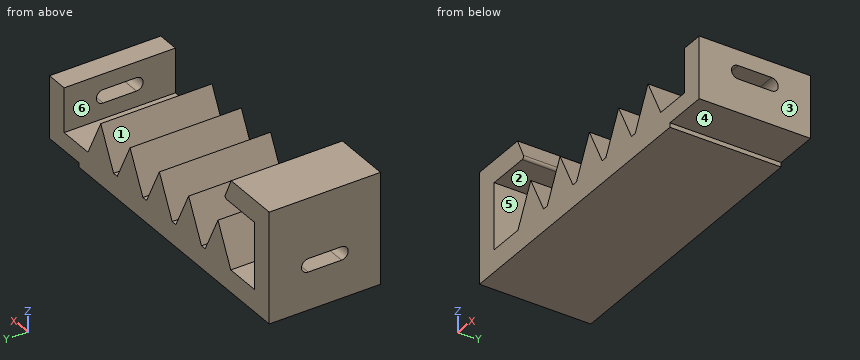
```python
from build123d import *

# Parameters (mm, degrees)
PAD028_DEPTH    = 2.5
POCKET033_DEPTH = 2


with BuildPart() as part:
    # Sketch063 → Pad028 (new body, symmetric)
    with BuildSketch(Plane.XZ):
        with BuildLine():
            Line((-7.5, 0), (-7.5, 5))
            Line((-7.5, 5), (-4.89997, 5))
            Line((-4.89997, 5), (-4.5, 4.142262))
            ThreePointArc((-4.590631, 4), (-4.506292, 4.04627), (-4.5, 4.142262))
            Line((-4.590631, 4), (-6.5, 4))
            Line((-6.5, 4), (-6.5, 1))
            Line((-6.5, 1), (-5, 1))
            Line((-4.875, 1), (-5, 1))
            Line((-4.875, 1), (-4, 2.75))
            Line((-4, 2.75), (-3.125, 1))
            Line((-3.125, 1), (-2.875, 1))
            Line((-2.875, 1), (-2, 2.75))
            Line((-2, 2.75), (-1.125, 1))
            Line((-1.125, 1), (-0.875, 1))
            Line((-0.875, 1), (0, 2.75))
            Line((0, 2.75), (0.875, 1))
            Line((0.875, 1), (1.125, 1))
            Line((1.125, 1), (2, 2.75))
            Line((2, 2.75), (2.875, 1))
            Line((2.875, 1), (3.125, 1))
            Line((3.125, 1), (4, 2.75))
            Line((4, 2.75), (4.875, 1))
            Line((4.875, 1), (5, 1))
            Line((5, 1), (6.5, 1))
            Line((6.5, 1), (6.5, 3))
            Line((6.5, 3), (7.5, 3))
            Line((7.5, 3), (7.5, 0.2))
            Line((5.5, 0.2), (7.5, 0.2))
            Line((5.5, 0), (5.5, 0.2))
            Line((5.5, 0), (-7.5, 0))
        make_face()
    extrude(amount=PAD028_DEPTH, both=True)

    # Sketch062 (on Face28 of Pad028) → Pocket033 (cut)
    with BuildSketch(Plane(origin=(7.5, 0, 0), x_dir=(0, 0, 1), z_dir=(1, 0, 0))):
        with BuildLine():
            ThreePointArc((2.3, 0.75), (2, 1.05), (1.7, 0.75))
            Line((1.7, 0.75), (1.7, -0.75))
            ThreePointArc((1.7, -0.75), (2, -1.05), (2.3, -0.75))
            Line((2.3, 0.75), (2.3, -0.75))
        make_face()
    pocket033 = extrude(amount=-POCKET033_DEPTH, mode=Mode.SUBTRACT)

    # Mirrored003: Pocket033 across YZ
    add(pocket033.mirror(Plane.YZ), mode=Mode.SUBTRACT)


solid = part.part
```
Can you work these out from the model? Positions are in its coordinate system, mm. Face numbers are marked on the shaded views. A direction names the side the tool comes from. Give positions to 0.01 mm unless a question says otherwise; leave off trailing zeros. Loops run counter-clockwise (first coordinate to the right, second up) from the corner with the lowest first, then second, coordinate; pieces in that order, holes last. Notation, with made-up numbers: M -34.75,-35 L 22.25,-35 A24 ccw 22.25,-14 Z; hole C 2,65.5 d4. An arc over 180 degrees is marked long. One line per question, with ' | ' between items. Start each with the question number.
Q1. If we section it at B-B (z = 1.4): Please give me the cut outline in (x, y) (3 decimals), plus the area to 4 significant figures.
Q2. If I drill on line 1 (Z direction, x = -5, y = 1.3); line 2 (Z direction, x = 6.75, y = 0.05); line 3 (X direction, y = 0.8, z = 3.7), over which ranges is the centre line in solid material (lowest first)? Write a range as from..to.
Q3. If we section it at A-A (x = -6.25): Please give me the cut outline in (y, z), plus the area to 3 significant figures.
Q4. For the marked faces 4, 5 and 6, which set-ups out of +Z, -Z, +X, -X, +Y, -Y let a thin tool reach every point of the face, with its end or its side?
Q5. For pin 1 Ø1.5 at (y, z) = (-0.5, 2) entering from +X; pin 2 Ø1.1 at (x, y) = (7, 0) entering from -Z, each with a flat end and sliding along its axis, tell me the tip position at first contact or that it passes through.
Q6. If we section it at C-C (y = 0.3): State how many separate pieces and enclosed holes the cut face has, plus the area to 3 significant figures.
Q7. If we mould it in two halves opening along X, with no side actions, what happens to the marked faces 1, 2 and 3? For each: +X half, -X half, draft (parallel to the pull), parting line (faces both ways), or undercut.
Computed:
1) outline: M -7.5,-2.5 L -6.5,-2.5 L -6.5,2.5 L -7.5,2.5 Z; M -4.675,-2.5 L -3.325,-2.5 L -3.325,2.5 L -4.675,2.5 Z; M -2.675,-2.5 L -1.325,-2.5 L -1.325,2.5 L -2.675,2.5 Z; M -0.675,-2.5 L 0.675,-2.5 L 0.675,2.5 L -0.675,2.5 Z; M 1.325,-2.5 L 2.675,-2.5 L 2.675,2.5 L 1.325,2.5 Z; M 3.325,-2.5 L 4.675,-2.5 L 4.675,2.5 L 3.325,2.5 Z; M 6.5,-2.5 L 7.5,-2.5 L 7.5,2.5 L 6.5,2.5 Z | area: 43.75 mm²
2) line 1: z = 0..1, 4..5 | line 2: z = 0.2..1.7, 2.3..3 | line 3: x = -7.5..-6.5
3) outline: M -2.5,0 L 2.5,0 L 2.5,1 L -2.5,1 Z; M -2.5,4 L 2.5,4 L 2.5,5 L -2.5,5 Z | area: 10.0 mm²
4) face 4: -Z, +X, +Y, -Y | face 5: +Y, -Y | face 6: +Z, +Y, -Y
5) pin 1: stops at x = 7.5 | pin 2: stops at z = 0.2
6) separate pieces: 3 | enclosed holes: 0 | area: 28.9 mm²
7) face 1: undercut | face 2: draft | face 3: +X half
